Answer from the drawing. Dimensions are ordinates in mm from the lowest x, y and z of the part. A direction names the side the tool comes from. Coordinates: 2 decimals unless noted, no trailing zeros. Order: outer loops, then holes, each group sorted by start corner. A loop starts at its lowest first (then second) coordinate and runs counter-clockwise, first axis right, second up.
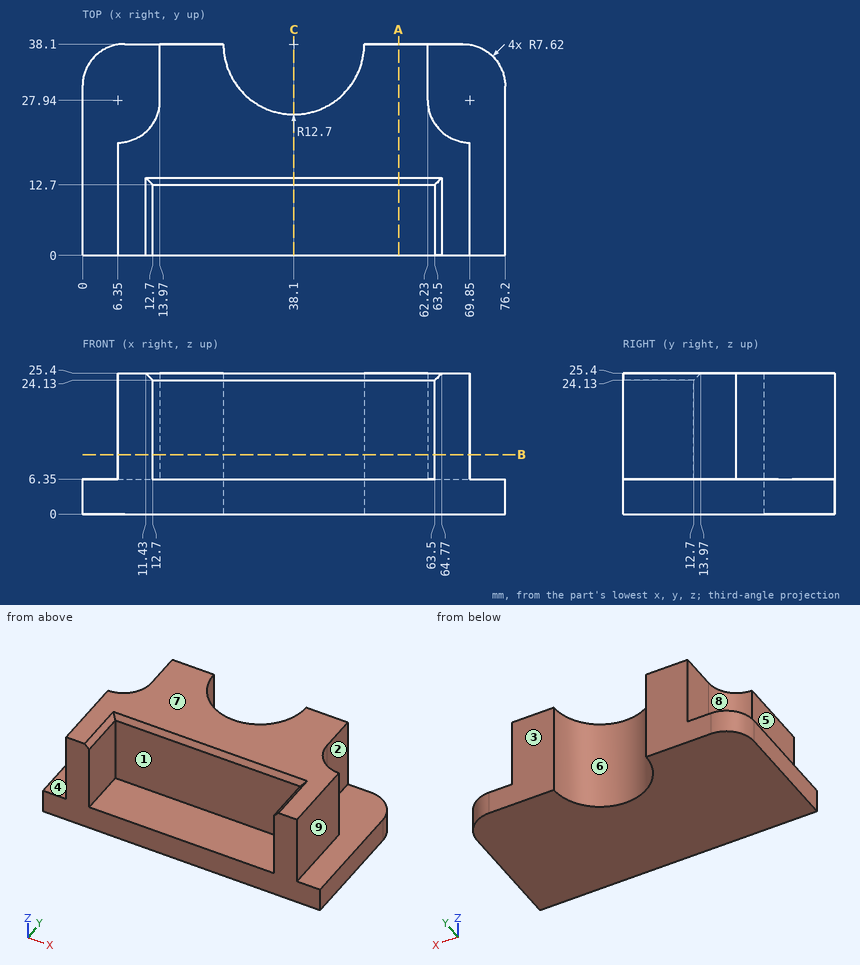
1. Consider probe 1 along X at (y, z) = (3, 15.5); probe 2 along X at (y, z) = (17.5, 17); probe 3 along Z at (x, y) = (71.5, 13). Determine where each line is inside the solid, lowest interval first.
2. The part is cut by section A-A (x = 57). Determine the outline of the cut face in (y, z).
3. The mould has two halves that part along X. Classify the marked faces 6, 7, 8 and 9: released by +X, released by -X, zero draft, split by the parting line, or undercut.
4. For the marked faces 1, 2, 3, 4 and 5, determine the directions among +Z, -Z, +X, -X, +Y, -Y from which every point of the face is accessible in a straight line to the end or side of a thin tool.
5. The part is cut by section C-C (x = 38.1). Determine the outline of the cut face in (y, z), plus the area to 3 significant figures.
6. The part is cut by section B-B (z = 10.75). Determine the outline of the cut face in (x, y).
7. Flat-ended cylindrical pins translate along their axes: pin 1 (11 mm diameter, centred on y = 30.5, z = 15.5, fed in from +X); pin 2 (1 mm diameter, centred on x = 48, y = 10, fed in from +Z); pin 3 (10 mm diameter, centred on x = 58, z = 19, fed in from -Y). Find the tip coordinate at first contact, or state that the pin passes through.
Worked out:
1. probe 1: x = 6.35 to 12.7, 63.5 to 69.85
1. probe 2: x = 6.35 to 69.85
1. probe 3: z = 0 to 6.35
2. outline: (0, 0) - (38.1, 0) - (38.1, 25.4) - (13.97, 25.4) - (12.7, 24.13) - (12.7, 6.35) - (0, 6.35) - close
3. face 6: undercut
3. face 7: zero draft
3. face 8: released by -X
3. face 9: released by +X
4. face 1: +Z, -Y
4. face 2: +Z, +X, +Y
4. face 3: +Z, -Z, +X, -X, +Y
4. face 4: +Z, -X, +Y
4. face 5: +Z, -X, +Y, -Y
5. outline: (0, 0) - (25.4, 0) - (25.4, 25.4) - (13.97, 25.4) - (12.7, 24.13) - (12.7, 6.35) - (0, 6.35) - close
5. area: 402 mm2
6. outline: (6.35, 0) - (12.7, 0) - (12.7, 12.7) - (63.5, 12.7) - (63.5, 0) - (69.85, 0) - (69.85, 20.32) arc R7.62 cw to (62.23, 27.94) - (62.23, 38.1) - (50.8, 38.1) arc R12.7 cw to (25.4, 38.1) - (13.97, 38.1) - (13.97, 27.94) arc R7.62 cw to (6.35, 20.32) - close
7. pin 1: stops at x = 62.82
7. pin 2: stops at z = 6.35
7. pin 3: stops at y = 12.7
